```python
from build123d import *

# Parameters (mm, degrees)
BASE_SKETCH_R       = 1.6
BASE_SKETCH_W       = 25
BASE_SKETCH_H       = 5
BASE_SKETCH_W_2     = 5
BASE_SKETCH_H_2     = 15
BASE_SKETCH_W_3     = 19
BASE_SKETCH_W_4     = 22
BASE_SKETCH_W_5     = 4.5
BASE_SKETCH_H_3     = 11.5
BASE_SKETCH_H_4     = 19
BASE_SKETCH_H_5     = 18.5
BOSS_EXTRUDE1_DEPTH = 2
BOSS_EXTRUDE2_START = 2
SKETCH1_7_R         = 1.6
BOSS_EXTRUDE2_DEPTH = 5
FILLET1_R           = 2


with BuildPart() as part:
    # Base_Sketch → Boss-Extrude1 (new body)
    # profile 1 of 47: a face of its own
    with BuildSketch(Plane.XY):
        Polygon((-46.5, -43.25), (-46.5, -47.75), (46.5, -47.75), (46.5, -43.25), (28, -43.25), (23, -43.25), (4, -43.25), (-1, -43.25), (-20, -43.25), (-25, -43.25), align=None)
    # profile 2 of 47: a face of its own
    with BuildSketch(Plane.XY):
        Polygon((-50, -39.75), (-54.5, -39.75), (-54.5, -47.75), (-46.5, -47.75), (-46.5, -43.25), (-50, -43.25), align=None)
        with Locations((-51.5, -44.75)):
            Circle(BASE_SKETCH_R, mode=Mode.SUBTRACT)
    # profile 3 of 47: a face of its own
    with BuildSketch(Plane.XY):
        Polygon((-50, 39.75), (-54.5, 39.75), (-54.5, -39.75), (-50, -39.75), (-50, -28.25), (-50, -23.25), (-50, -4.25), (-50, 0.75), (-50, 19.75), (-50, 24.75), align=None)
    # profile 4 of 47: a face of its own
    with BuildSketch(Plane.XY):
        with Locations((-37.5, -25.75)):
            Rectangle(BASE_SKETCH_W, BASE_SKETCH_H)
    # profile 5 of 47: a face of its own
    with BuildSketch(Plane.XY):
        with Locations((-22.5, -25.75)):
            Rectangle(BASE_SKETCH_W_2, BASE_SKETCH_H)
    # profile 6 of 47: a face of its own
    with BuildSketch(Plane.XY):
        with Locations((-22.5, -35.75)):
            Rectangle(BASE_SKETCH_W_2, BASE_SKETCH_H_2)
    # profile 7 of 47: a face of its own
    with BuildSketch(Plane.XY):
        with Locations((-10.5, -25.75)):
            Rectangle(BASE_SKETCH_W_3, BASE_SKETCH_H)
    # profile 8 of 47: a face of its own
    with BuildSketch(Plane.XY):
        with Locations((1.5, -25.75)):
            Rectangle(BASE_SKETCH_W_2, BASE_SKETCH_H)
    # profile 9 of 47: a face of its own
    with BuildSketch(Plane.XY):
        with Locations((1.5, -35.75)):
            Rectangle(BASE_SKETCH_W_2, BASE_SKETCH_H_2)
    # profile 10 of 47: a face of its own
    with BuildSketch(Plane.XY):
        with Locations((13.5, -25.75)):
            Rectangle(BASE_SKETCH_W_3, BASE_SKETCH_H)
    # profile 11 of 47: a face of its own
    with BuildSketch(Plane.XY):
        with Locations((25.5, -25.75)):
            Rectangle(BASE_SKETCH_W_2, BASE_SKETCH_H)
    # profile 12 of 47: a face of its own
    with BuildSketch(Plane.XY):
        with Locations((25.5, -35.75)):
            Rectangle(BASE_SKETCH_W_2, BASE_SKETCH_H_2)
    # profile 13 of 47: a face of its own
    with BuildSketch(Plane.XY):
        with Locations((39, -25.75)):
            Rectangle(BASE_SKETCH_W_4, BASE_SKETCH_H)
    # profile 14 of 47: a face of its own
    with BuildSketch(Plane.XY):
        with Locations((52.25, -25.75)):
            Rectangle(BASE_SKETCH_W_5, BASE_SKETCH_H)
    # profile 15 of 47: a face of its own
    with BuildSketch(Plane.XY):
        with Locations((52.25, -34)):
            Rectangle(BASE_SKETCH_W_5, BASE_SKETCH_H_3)
    # profile 16 of 47: a face of its own
    with BuildSketch(Plane.XY):
        Polygon((46.5, -43.25), (46.5, -47.75), (54.5, -47.75), (54.5, -39.75), (50, -39.75), (50, -43.25), align=None)
        with Locations((51.5, -44.75)):
            Circle(BASE_SKETCH_R, mode=Mode.SUBTRACT)
    # profile 17 of 47: a face of its own
    with BuildSketch(Plane.XY):
        with Locations((52.25, -13.75)):
            Rectangle(BASE_SKETCH_W_5, BASE_SKETCH_H_4)
    # profile 18 of 47: a face of its own
    with BuildSketch(Plane.XY):
        with Locations((52.25, -1.75)):
            Rectangle(BASE_SKETCH_W_5, BASE_SKETCH_H)
    # profile 19 of 47: a face of its own
    with BuildSketch(Plane.XY):
        with Locations((39, -1.75)):
            Rectangle(BASE_SKETCH_W_4, BASE_SKETCH_H)
    # profile 20 of 47: a face of its own
    with BuildSketch(Plane.XY):
        with Locations((25.5, -1.75)):
            Rectangle(BASE_SKETCH_W_2, BASE_SKETCH_H)
    # profile 21 of 47: a face of its own
    with BuildSketch(Plane.XY):
        with Locations((25.5, -13.75)):
            Rectangle(BASE_SKETCH_W_2, BASE_SKETCH_H_4)
    # profile 22 of 47: a face of its own
    with BuildSketch(Plane.XY):
        with Locations((25.5, 10.25)):
            Rectangle(BASE_SKETCH_W_2, BASE_SKETCH_H_4)
    # profile 23 of 47: a face of its own
    with BuildSketch(Plane.XY):
        with Locations((13.5, -1.75)):
            Rectangle(BASE_SKETCH_W_3, BASE_SKETCH_H)
    # profile 24 of 47: a face of its own
    with BuildSketch(Plane.XY):
        with Locations((1.5, -1.75)):
            Rectangle(BASE_SKETCH_W_2, BASE_SKETCH_H)
    # profile 25 of 47: a face of its own
    with BuildSketch(Plane.XY):
        with Locations((1.5, -13.75)):
            Rectangle(BASE_SKETCH_W_2, BASE_SKETCH_H_4)
    # profile 26 of 47: a face of its own
    with BuildSketch(Plane.XY):
        with Locations((52.25, 10.25)):
            Rectangle(BASE_SKETCH_W_5, BASE_SKETCH_H_4)
    # profile 27 of 47: a face of its own
    with BuildSketch(Plane.XY):
        with Locations((52.25, 22.25)):
            Rectangle(BASE_SKETCH_W_5, BASE_SKETCH_H)
    # profile 28 of 47: a face of its own
    with BuildSketch(Plane.XY):
        with Locations((52.25, 32.25)):
            Rectangle(BASE_SKETCH_W_5, BASE_SKETCH_H_2)
    # profile 29 of 47: a face of its own
    with BuildSketch(Plane.XY):
        Polygon((54.5, 47.75), (46.5, 47.75), (46.5, 43.25), (50, 43.25), (50, 39.75), (54.5, 39.75), align=None)
        with Locations((51.5, 44.75)):
            Circle(BASE_SKETCH_R, mode=Mode.SUBTRACT)
    # profile 30 of 47: a face of its own
    with BuildSketch(Plane.XY):
        Polygon((46.5, 47.75), (-46.5, 47.75), (-46.5, 43.25), (-25, 43.25), (-20, 43.25), (-1, 43.25), (4, 43.25), (23, 43.25), (28, 43.25), (46.5, 43.25), align=None)
    # profile 31 of 47: a face of its own
    with BuildSketch(Plane.XY):
        with Locations((39, 22.25)):
            Rectangle(BASE_SKETCH_W_4, BASE_SKETCH_H)
    # profile 32 of 47: a face of its own
    with BuildSketch(Plane.XY):
        with Locations((25.5, 34)):
            Rectangle(BASE_SKETCH_W_2, BASE_SKETCH_H_5)
    # profile 33 of 47: a face of its own
    with BuildSketch(Plane.XY):
        with Locations((25.5, 22.25)):
            Rectangle(BASE_SKETCH_W_2, BASE_SKETCH_H)
    # profile 34 of 47: a face of its own
    with BuildSketch(Plane.XY):
        with Locations((13.5, 22.25)):
            Rectangle(BASE_SKETCH_W_3, BASE_SKETCH_H)
    # profile 35 of 47: a face of its own
    with BuildSketch(Plane.XY):
        with Locations((1.5, 22.25)):
            Rectangle(BASE_SKETCH_W_2, BASE_SKETCH_H)
    # profile 36 of 47: a face of its own
    with BuildSketch(Plane.XY):
        with Locations((1.5, 34)):
            Rectangle(BASE_SKETCH_W_2, BASE_SKETCH_H_5)
    # profile 37 of 47: a face of its own
    with BuildSketch(Plane.XY):
        with Locations((1.5, 10.25)):
            Rectangle(BASE_SKETCH_W_2, BASE_SKETCH_H_4)
    # profile 38 of 47: a face of its own
    with BuildSketch(Plane.XY):
        with Locations((-10.5, 22.25)):
            Rectangle(BASE_SKETCH_W_3, BASE_SKETCH_H)
    # profile 39 of 47: a face of its own
    with BuildSketch(Plane.XY):
        with Locations((-10.5, -1.75)):
            Rectangle(BASE_SKETCH_W_3, BASE_SKETCH_H)
    # profile 40 of 47: a face of its own
    with BuildSketch(Plane.XY):
        with Locations((-22.5, -1.75)):
            Rectangle(BASE_SKETCH_W_2, BASE_SKETCH_H)
    # profile 41 of 47: a face of its own
    with BuildSketch(Plane.XY):
        Polygon((-46.5, 47.75), (-54.5, 47.75), (-54.5, 39.75), (-50, 39.75), (-50, 43.25), (-46.5, 43.25), align=None)
        with Locations((-51.5, 44.75)):
            Circle(BASE_SKETCH_R, mode=Mode.SUBTRACT)
    # profile 42 of 47: a face of its own
    with BuildSketch(Plane.XY):
        with Locations((-37.5, 22.25)):
            Rectangle(BASE_SKETCH_W, BASE_SKETCH_H)
    # profile 43 of 47: a face of its own
    with BuildSketch(Plane.XY):
        with Locations((-22.5, 22.25)):
            Rectangle(BASE_SKETCH_W_2, BASE_SKETCH_H)
    # profile 44 of 47: a face of its own
    with BuildSketch(Plane.XY):
        with Locations((-22.5, 34)):
            Rectangle(BASE_SKETCH_W_2, BASE_SKETCH_H_5)
    # profile 45 of 47: a face of its own
    with BuildSketch(Plane.XY):
        with Locations((-22.5, 10.25)):
            Rectangle(BASE_SKETCH_W_2, BASE_SKETCH_H_4)
    # profile 46 of 47: a face of its own
    with BuildSketch(Plane.XY):
        with Locations((-37.5, -1.75)):
            Rectangle(BASE_SKETCH_W, BASE_SKETCH_H)
    # profile 47 of 47: a face of its own
    with BuildSketch(Plane.XY):
        with Locations((-22.5, -13.75)):
            Rectangle(BASE_SKETCH_W_2, BASE_SKETCH_H_4)
    extrude(amount=BOSS_EXTRUDE1_DEPTH)

    # Sketch1<7> → Boss-Extrude2 (add)
    # profile 1 of 4: a face of its own
    with BuildSketch(Plane.XY.offset(BOSS_EXTRUDE2_START)):
        Polygon((-46.5, 47.75), (-54.5, 47.75), (-54.5, 39.75), (-50, 39.75), (-50, 43.25), (-46.5, 43.25), align=None)
        with Locations((-51.5, 44.75)):
            Circle(SKETCH1_7_R, mode=Mode.SUBTRACT)
    # profile 2 of 4: a face of its own
    with BuildSketch(Plane.XY.offset(BOSS_EXTRUDE2_START)):
        Polygon((54.5, 47.75), (46.5, 47.75), (46.5, 43.25), (50, 43.25), (50, 39.75), (54.5, 39.75), align=None)
        with Locations((51.5, 44.75)):
            Circle(SKETCH1_7_R, mode=Mode.SUBTRACT)
    # profile 3 of 4: a face of its own
    with BuildSketch(Plane.XY.offset(BOSS_EXTRUDE2_START)):
        Polygon((-50, -39.75), (-54.5, -39.75), (-54.5, -47.75), (-46.5, -47.75), (-46.5, -43.25), (-50, -43.25), align=None)
        with Locations((-51.5, -44.75)):
            Circle(SKETCH1_7_R, mode=Mode.SUBTRACT)
    # profile 4 of 4: a face of its own
    with BuildSketch(Plane.XY.offset(BOSS_EXTRUDE2_START)):
        Polygon((46.5, -43.25), (46.5, -47.75), (54.5, -47.75), (54.5, -39.75), (50, -39.75), (50, -43.25), align=None)
        with Locations((51.5, -44.75)):
            Circle(SKETCH1_7_R, mode=Mode.SUBTRACT)
    extrude(amount=BOSS_EXTRUDE2_DEPTH)

    # Fillet1
    fillet1_edges = [part.edges().sort_by_distance(p)[0] for p in [
        (-50, -43.25, 3.5),
        (50, -43.25, 3.5),
        (-50, 43.25, 3.5),
        (50, 43.25, 3.5),
        (54.5, -47.75, 3.5),
        (-54.5, -47.75, 3.5),
        (-54.5, 47.75, 3.5),
        (54.5, 47.75, 3.5),
        (-46.5, 45.5, 2),
        (-52.25, 39.75, 2),
        (52.25, 39.75, 2),
        (46.5, 45.5, 2),
        (-52.25, -39.75, 2),
        (-46.5, -45.5, 2),
        (46.5, -45.5, 2),
        (52.25, -39.75, 2),
    ]]
    fillet(fillet1_edges, radius=FILLET1_R)


solid = part.part
```
Design review of the part built by this model. Coordinates are the model's own, in mm. A direction names the side the tool comes from. Round coordinates to 2 decimals unless told otherwise and drop trailing zeros. Write each loop counter-clockwise with the first axis right and the second up, starting at its lowest first coordinate (ties: lowest second). Pieces come first, ordered by that corner, then holes. Notation, with made-up numbers: (77.25, 28) -> (109.25, 28) arc R12 ccw to (109.25, 39) -> close; hole circle Ø4 at (-35, 87). An arc over 180 degrees is marked (long way). Write item = value, one per line. Start each with the question number.
1) Mouldability with a two-part tool opening along X and no side actions: class faces 1 (the face through (-39, 43.25, 1)), 2 (the face through (12, 47.75, 1)) as +X half, -X half, draft (parallel to the pull), parting line (faces both ways), or undercut.
2) Clearance check with flat-ended pins moving along their axes: pin 1 (5 mm diameter, centred on x = 51.5, y = -44.75, fed in from -Z); pin 2 (10 mm diameter, centred on x = 35.5, y = 30.5, fed in from +Z). State where each tip first meets the part, or that it passes through.
3) Take a section at B-B, the plane x = 39.5. State the section outline as (y, z) points, plus the area to 3 significant figures.
4) Wall thickness on probe 1 along Y at (x, z) = (-4, 1); probe 2 along Y at (x, z) = (51.5, 4); probe 3 along X at (y, z) = (-42.5, 1.5): over which ranges is each line inside the solid? List them lowest first. Write a range as from..to.
5) Take a section at A-A, the plane y = 15.5. State the section outline as (x, z) points, plus the area to 3 significant figures.
6) Take a section at C-C, the plane x = -23.5. State the section outline as (y, z) points, plus the area to 3 significant figures.
7) Tool access review of faces 3 (the face through (46.5, 46, 5)), 4 (the face through (-12, -47.75, 1)), 5 (the face through (-52, -39.75, 5)), 6 (the face through (-50, -36, 1)), 7 (the face through (-51, 43, 7)): name each direction out of +Z, -Z, +X, -X, +Y, -Y from which nothing blocks a thin tool from reaching the whole face with its end or side.
Results list:
q1.face_1 = undercut
q1.face_2 = draft
q2.pin_1 = 0
q2.pin_2 = through
q3.outline = (-47.75, 0) -> (-43.25, 0) -> (-43.25, 2) -> (-47.75, 2) -> close; (-28.25, 0) -> (-23.25, 0) -> (-23.25, 2) -> (-28.25, 2) -> close; (-4.25, 0) -> (0.75, 0) -> (0.75, 2) -> (-4.25, 2) -> close; (19.75, 0) -> (24.75, 0) -> (24.75, 2) -> (19.75, 2) -> close; (43.25, 0) -> (47.75, 0) -> (47.75, 2) -> (43.25, 2) -> close
q3.area = 48.0 mm²
q4.probe_1 = -47.75..-43.25, -28.25..-23.25, -4.25..0.75, 19.75..24.75, 43.25..47.75
q4.probe_2 = -47.75..-46.35, -43.15..-39.75, 39.75..43.15, 46.35..47.75
q4.probe_3 = -54.5..-49.56, -25..-20, -1..4, 23..28, 49.56..54.5
q5.outline = (-54.5, 0) -> (-50, 0) -> (-50, 2) -> (-54.5, 2) -> close; (-25, 0) -> (-20, 0) -> (-20, 2) -> (-25, 2) -> close; (-1, 0) -> (4, 0) -> (4, 2) -> (-1, 2) -> close; (23, 0) -> (28, 0) -> (28, 2) -> (23, 2) -> close; (50, 0) -> (54.5, 0) -> (54.5, 2) -> (50, 2) -> close
q5.area = 48.0 mm²
q6.outline = (-47.75, 0) -> (47.75, 0) -> (47.75, 2) -> (-47.75, 2) -> close
q6.area = 191 mm²
q7.face_3 = +Z, +Y, -Y
q7.face_4 = +Z, -Z, +X, -X, -Y
q7.face_5 = +Z, +X, -X
q7.face_6 = +Z, -Z
q7.face_7 = +Z, +X, -X, +Y, -Y
